Input: part model. Units: mm. Frame: model coordinates. A direction names the side the tool comes from. Coordinates: 2 decimals unless noted, no trailing zeros. Write each loop counter-clockwise with the first axis right and the second up, starting at its lowest first coordinate (ties: lowest second). Pieces come first, ordered by that corner, then holes. Notation, with made-up numbers: (20, 34) -> (48, 34) arc R14 ccw to (48, 51) -> close; hole circle Ø5 at (-13.5, 41). An arc over 180 degrees is marked (long way). Use one line per item in the form item = value. Start each with the question number.
(1) Ray query, line 1 along Y through (x, z) = (0, -3.75); line 2 along Y through (x, z) = (2.25, -0.25); line 3 along X through (y, z) = (4, -0.25). Return the intervals inside material, ascending.
(2) Cut plane A-A on z = -4.75. Return the cut outline in (x, y), plus the area to 3 significant figures.
(3) Set-up query: faces 5 (the face through (0, -6, -3)), 6 (the face through (1.89, -0.76, -3)), 7 (the face through (-1.054, -3.766, -5.168)), 8 (the face through (2, 3, -1)). Return all of +Z, -Z, +X, -X, +Y, -Y with unobstructed straight access to the full face (end or side cutting, diameter ignored); none if empty.
(4) Pull-direction query (X, two-part tool) for faces 1 (the face through (1.89, -3.74, -3)), 2 (the face through (3.71, 5.23, -1.43)), 3 (the face through (0.019, 7.193, -4.774)), 4 (the face through (-1.054, 5.234, -5.168)); classes: released by +X, released by -X, zero draft, split by the parting line, or undercut.
(5) Cut plane D-D on z = -4. Return the cut outline in (x, y), plus the area to 3 significant figures.
(6) First-contact query: pin 1 (1.5 mm diameter, centred on x = 2.5, z = -2, fed in from -Y); pin 2 (2 mm diameter, centred on x = 1, z = -3, fed in from -Y); pin 3 (2.5 mm diameter, centred on x = 2.5, z = -1.5, fed in from +Y). Flat tips, straight axial feed; report the tip coordinate or a pass-through.
(7) Cut plane C-C on y = -6.25. Return the cut outline in (x, z).
(8) Cut plane B-B on x = 0.25. Return the cut outline in (y, z).
```python
from build123d import *

# Parameters (mm, degrees)
SKETCH1_W           = 15
SKETCH1_H           = 30
BOSS_EXTRUDE1_DEPTH = 7
CUT_EXTRUDE1_START  = -0.3
CUT_EXTRUDE1_DEPTH  = 2.1
CUT_EXTRUDE4_DEPTH  = 2.7
BOSS_EXTRUDE2_DEPTH = 24.556743
CUT_EXTRUDE2_DEPTH  = 27.627139608
CUT_EXTRUDE3_DEPTH  = 27.401285317
SKETCH13_W          = 10
SKETCH13_H          = 20
BOSS_EXTRUDE3_DEPTH = 7
SKETCH14_W          = 3.65
SKETCH14_H          = 19.113486034
CUT_EXTRUDE5_DEPTH  = 13.592908206


with BuildPart() as part:
    # Sketch1 → Boss-Extrude1 (new body)
    with BuildSketch(Plane.XY):
        Rectangle(SKETCH1_W, SKETCH1_H)
    extrude(amount=-BOSS_EXTRUDE1_DEPTH)

    # Sketch8 → Cut-Extrude1 (cut)
    with BuildSketch(Plane(origin=(1.35, 0, 0), x_dir=(0, 0, -1), z_dir=(1, 0, 0)).offset(CUT_EXTRUDE1_START)):
        Polygon((6.5, -4.716092451), (6.5, -2.783907549), (3, -2.600480321), (3, -1.899519679), (6.5, -1.716092451), (6.5, 0.216092451), (3, 0.399519679), (3, 1.100480321), (6.5, 1.283907549), (6.5, 3.216092451), (3, 3.399519679), (3, 4.100480321), (6.5, 4.283907549), (6.5, 6.216092451), (3, 6.399519679), (3, 7.100480321), (6.5, 7.283907549), (6.5, 9.216092451), (0, 9.556743017), (0, -9.556743017), (6.5, -9.216092451), (6.5, -7.283907549), (3, -7.100480321), (3, -4.899519679), align=None)
    extrude(amount=-CUT_EXTRUDE1_DEPTH, mode=Mode.SUBTRACT)

    # Sketch7 → Cut-Extrude4 (cut)
    with BuildSketch(Plane(origin=(1.35, 0, 0), x_dir=(0, 0, -1), z_dir=(1, 0, 0))):
        Polygon((3, 4.100480321), (0, 4.100480321), (0, 6.399519679), (3, 6.399519679), (6.5, 6.216092451), (6.5, 4.283907549), align=None)
        Polygon((3, 1.100480321), (0, 1.100480321), (0, 3.399519679), (3, 3.399519679), (6.5, 3.216092451), (6.5, 1.283907549), align=None)
        Polygon((3, -1.899519679), (0, -1.899519679), (0, 0.399519679), (3, 0.399519679), (6.5, 0.216092451), (6.5, -1.716092451), align=None)
        Polygon((3, -4.899519679), (0, -4.899519679), (0, -2.600480321), (3, -2.600480321), (6.5, -2.783907549), (6.5, -4.716092451), align=None)
        Polygon((3, -7.100480321), (0, -7.100480321), (0, -9.556743017), (6.5, -9.216092451), (6.5, -7.283907549), align=None)
        Polygon((3, 7.100480321), (0, 7.100480321), (0, 9.556743017), (6.5, 9.216092451), (6.5, 7.283907549), align=None)
    extrude(amount=-CUT_EXTRUDE4_DEPTH, mode=Mode.SUBTRACT)

    # Sketch10 → Boss-Extrude2 (add)
    with BuildSketch(Plane(origin=(0, -9.556743017, 0), x_dir=(1, 0, 0), z_dir=(0, 1, 0))):
        with BuildLine():
            Line((1.35, 3.599507213), (1.35, 6.5))
            ThreePointArc((1.35, 6.5), (1.052815056, 5.148153684), (1.246508191, 3.777646361))
            ThreePointArc((1.246508191, 3.777646361), (1.288979573, 3.683188656), (1.35, 3.599507213))
        make_face()
        with BuildLine():
            Line((-1.35, 3.599507213), (-1.35, 6.5))
            ThreePointArc((-1.35, 6.5), (-1.052815056, 5.148153684), (-1.246508191, 3.777646361))
            ThreePointArc((-1.246508191, 3.777646361), (-1.288979573, 3.683188656), (-1.35, 3.599507213))
        make_face()
    extrude(amount=BOSS_EXTRUDE2_DEPTH)

    # Sketch12 → Cut-Extrude2 (cut, through all)
    with BuildSketch(Plane(origin=(3.10411931, 9.156194078, -3.38952842), x_dir=(0, -1, 0), z_dir=(0.669702306213578, 0, 0.7426296661541438))):
        with BuildLine():
            Line((0.156194078, -1.612037756), (0.156194078, -5.06124645))
            Line((0.156194078, -5.06124645), (1.656194078, -5.06124645))
            Line((1.656194078, -5.06124645), (1.656194078, -1.612037756))
            ThreePointArc((1.656194078, -1.612037756), (0.906194078, -0.862037756), (0.156194078, -1.612037756))
        make_face()
        with BuildLine():
            Line((3.156194078, -1.612037756), (3.156194078, -5.06124645))
            Line((3.156194078, -5.06124645), (4.656194078, -5.06124645))
            Line((4.656194078, -5.06124645), (4.656194078, -1.612037756))
            ThreePointArc((4.656194078, -1.612037756), (3.906194078, -0.862037756), (3.156194078, -1.612037756))
        make_face()
        with BuildLine():
            Line((6.156194078, -1.612037756), (6.156194078, -5.06124645))
            Line((6.156194078, -5.06124645), (7.656194078, -5.06124645))
            Line((7.656194078, -5.06124645), (7.656194078, -1.612037756))
            ThreePointArc((7.656194078, -1.612037756), (6.906194078, -0.862037756), (6.156194078, -1.612037756))
        make_face()
        with BuildLine():
            Line((9.156194078, -1.612037756), (9.156194078, -5.06124645))
            Line((9.156194078, -5.06124645), (10.656194078, -5.06124645))
            Line((10.656194078, -5.06124645), (10.656194078, -1.612037756))
            ThreePointArc((10.656194078, -1.612037756), (9.906194078, -0.862037756), (9.156194078, -1.612037756))
        make_face()
        with BuildLine():
            Line((12.156194078, -1.612037756), (12.156194078, -5.06124645))
            Line((12.156194078, -5.06124645), (13.656194078, -5.06124645))
            Line((13.656194078, -5.06124645), (13.656194078, -1.612037756))
            ThreePointArc((13.656194078, -1.612037756), (12.906194078, -0.862037756), (12.156194078, -1.612037756))
        make_face()
        with BuildLine():
            Line((16.656194078, -1.612037756), (16.656194078, -5.06124645))
            Line((16.656194078, -5.06124645), (18.156194078, -5.06124645))
            Line((18.156194078, -5.06124645), (18.156194078, -1.612037756))
            ThreePointArc((18.156194078, -1.612037756), (17.406194078, -0.862037756), (16.656194078, -1.612037756))
        make_face()
    cut_extrude2 = extrude(amount=CUT_EXTRUDE2_DEPTH, mode=Mode.SUBTRACT)

    # Sketch11 → Cut-Extrude3 (cut, through all)
    with BuildSketch(Plane(origin=(2.212963711, 9.156194078, -4.377726578), x_dir=(0, -1, 0), z_dir=(0.6697023062135781, 0, 0.7426296661541438))):
        with BuildLine():
            Line((0.456194078, -2.362037756), (0.456194078, -1.612037756))
            ThreePointArc((0.456194078, -1.612037756), (0.906194078, -1.162037756), (1.356194078, -1.612037756))
            Line((1.356194078, -1.612037756), (1.356194078, -2.362037756))
            Line((1.356194078, -2.362037756), (0.456194078, -2.362037756))
        make_face()
        with BuildLine():
            Line((3.456194078, -1.612037756), (3.456194078, -2.362037756))
            Line((3.456194078, -2.362037756), (4.356194078, -2.362037756))
            Line((4.356194078, -2.362037756), (4.356194078, -1.612037756))
            ThreePointArc((4.356194078, -1.612037756), (3.906194078, -1.162037756), (3.456194078, -1.612037756))
        make_face()
        with BuildLine():
            Line((7.356194078, -1.612037756), (7.356194078, -2.362037756))
            Line((7.356194078, -2.362037756), (6.456194078, -2.362037756))
            Line((6.456194078, -2.362037756), (6.456194078, -1.612037756))
            ThreePointArc((6.456194078, -1.612037756), (6.906194078, -1.162037756), (7.356194078, -1.612037756))
        make_face()
        with BuildLine():
            Line((9.456194078, -1.612037756), (9.456194078, -2.362037756))
            Line((9.456194078, -2.362037756), (10.356194078, -2.362037756))
            Line((10.356194078, -2.362037756), (10.356194078, -1.612037756))
            ThreePointArc((10.356194078, -1.612037756), (9.906194078, -1.162037756), (9.456194078, -1.612037756))
        make_face()
        with BuildLine():
            Line((13.356194078, -1.612037756), (13.356194078, -2.362037756))
            Line((13.356194078, -2.362037756), (12.456194078, -2.362037756))
            Line((12.456194078, -2.362037756), (12.456194078, -1.612037756))
            ThreePointArc((12.456194078, -1.612037756), (12.906194078, -1.162037756), (13.356194078, -1.612037756))
        make_face()
        with BuildLine():
            Line((16.956194078, -1.612037756), (16.956194078, -2.362037756))
            Line((16.956194078, -2.362037756), (17.856194078, -2.362037756))
            Line((17.856194078, -2.362037756), (17.856194078, -1.612037756))
            ThreePointArc((17.856194078, -1.612037756), (17.406194078, -1.162037756), (16.956194078, -1.612037756))
        make_face()
    cut_extrude3 = extrude(amount=CUT_EXTRUDE3_DEPTH, mode=Mode.SUBTRACT)

    # Mirror1: Cut-Extrude2, Cut-Extrude3 across plane
    add(cut_extrude2.mirror(Plane(origin=(0, 0, 0), x_dir=(0, 0, 1), z_dir=(1, 0, 0))), mode=Mode.SUBTRACT)
    add(cut_extrude3.mirror(Plane(origin=(0, 0, 0), x_dir=(0, 0, 1), z_dir=(1, 0, 0))), mode=Mode.SUBTRACT)


with BuildPart() as body_2:
    # Sketch13 → Boss-Extrude3 (new body)
    with BuildSketch(Plane.XY):
        Rectangle(SKETCH13_W, SKETCH13_H)
    extrude(amount=-BOSS_EXTRUDE3_DEPTH)

    # Combine1: cut part
    add(part.part, mode=Mode.SUBTRACT)

    # Sketch14 → Cut-Extrude5 (cut, through all)
    with BuildSketch(Plane.XY):
        with Locations((-3.175, 0)):
            Rectangle(SKETCH14_W, SKETCH14_H)
    extrude(amount=-CUT_EXTRUDE5_DEPTH, mode=Mode.SUBTRACT)


solid = body_2.part
```
Values:
q1.line_1 = -9.36 to -7.14, -4.86 to -2.64, -1.86 to 0.36, 1.14 to 3.36, 4.14 to 6.36, 7.14 to 9.36
q1.line_2 = -9 to -7.5, -4.5 to -3, -1.5 to 0, 1.5 to 3, 4.5 to 6, 7.5 to 9
q1.line_3 = -1.05 to 1.05
q2.outline = (-1.06, -9.31) -> (1.06, -9.31) -> (1.06, -7.19) -> (-1.06, -7.19) -> close; (-1.06, -4.81) -> (1.06, -4.81) -> (1.06, -2.69) -> (-1.06, -2.69) -> close; (-1.06, -1.81) -> (1.06, -1.81) -> (1.06, 0.31) -> (-1.06, 0.31) -> close; (-1.06, 1.19) -> (1.06, 1.19) -> (1.06, 3.31) -> (-1.06, 3.31) -> close; (-1.06, 4.19) -> (1.06, 4.19) -> (1.06, 6.31) -> (-1.06, 6.31) -> close; (-1.06, 7.19) -> (1.06, 7.19) -> (1.06, 9.31) -> (-1.06, 9.31) -> close
q2.area = 26.9 mm2
q3.face_5 = -Z, +X, -X
q3.face_6 = -Z
q3.face_7 = -X, +Y, -Y
q3.face_8 = +Z, -Z, +X
q4.face_1 = undercut
q4.face_2 = released by +X
q4.face_3 = zero draft
q4.face_4 = released by -X
q5.outline = (-1.18, -9.35) -> (1.18, -9.35) -> (1.18, -7.15) -> (-1.18, -7.15) -> close; (-1.18, -4.85) -> (1.18, -4.85) -> (1.18, -2.65) -> (-1.18, -2.65) -> close; (-1.18, -1.85) -> (1.18, -1.85) -> (1.18, 0.35) -> (-1.18, 0.35) -> close; (-1.18, 1.15) -> (1.18, 1.15) -> (1.18, 3.35) -> (-1.18, 3.35) -> close; (-1.18, 4.15) -> (1.18, 4.15) -> (1.18, 6.35) -> (-1.18, 6.35) -> close; (-1.18, 7.15) -> (1.18, 7.15) -> (1.18, 9.35) -> (-1.18, 9.35) -> close
q5.area = 31.1 mm2
q6.pin_1 = -9
q6.pin_2 = -9.45
q6.pin_3 = 9.5
q7.outline = (-1.05, -3) -> (1.05, -3) -> (1.05, 0) -> (-1.05, 0) -> close
q8.outline = (-9.56, 0) -> (-9.22, -6.5) -> (-7.28, -6.5) -> (-7.1, -3) -> (-4.9, -3) -> (-4.72, -6.5) -> (-2.78, -6.5) -> (-2.6, -3) -> (-1.9, -3) -> (-1.72, -6.5) -> (0.22, -6.5) -> (0.4, -3) -> (1.1, -3) -> (1.28, -6.5) -> (3.22, -6.5) -> (3.4, -3) -> (4.1, -3) -> (4.28, -6.5) -> (6.22, -6.5) -> (6.4, -3) -> (7.1, -3) -> (7.28, -6.5) -> (9.22, -6.5) -> (9.56, 0) -> close
